For this review, use the dimensioned drawing (mm, ordinates from the lowest corner) and the shaded views. A direction names the side the tool comes from. Give positions to 0.01 mm unless a question says otherwise; leave off trailing zeros. Write each loop counter-clockwise with the first axis right and the second up, starting at its lowest first coordinate (ties: lowest second). Pieces come first, ordered by that corner, then holes. Notation, with made-up numbers: (-10, 62) -> (33, 62) arc R16 ccw to (33, 87) -> close; hole circle Ø4 at (61, 21). An arc over 180 degrees is marked (long way). Answer as CSV lines item,"result".
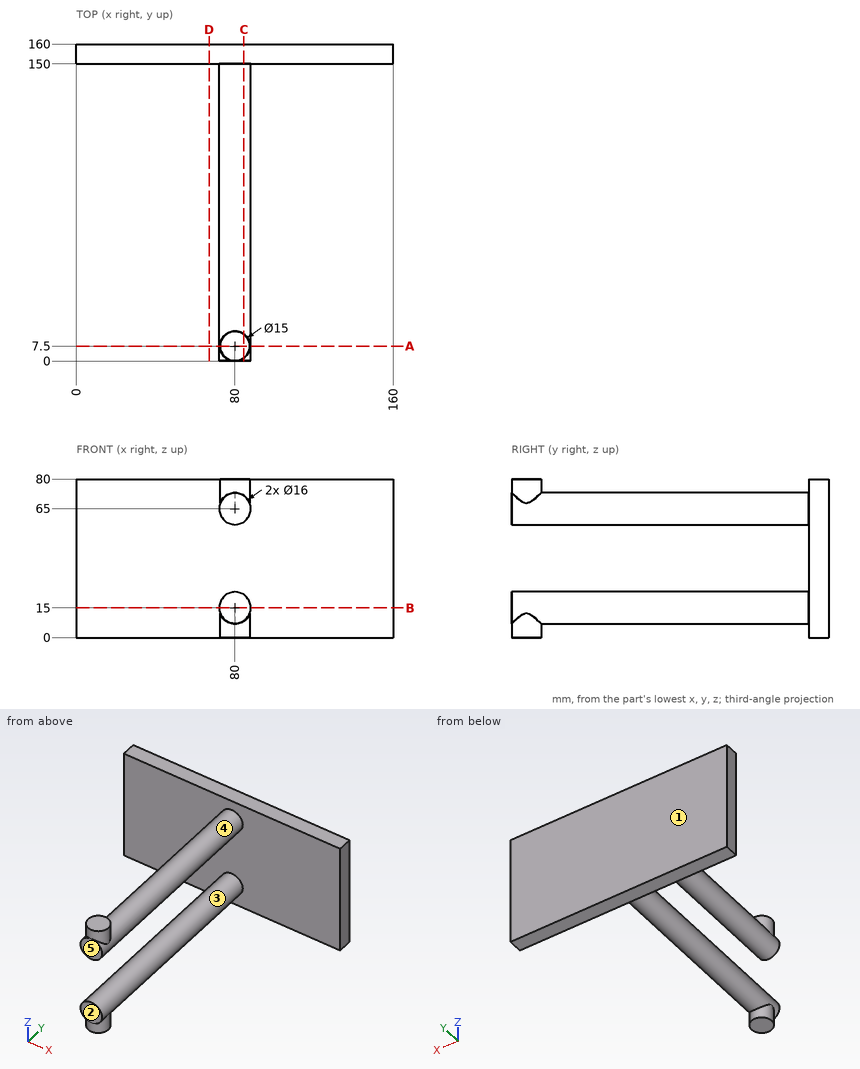
Q1. Clearance check with flat-ended pins moving along their axes: pin 1 (8 mm diameter, centred on x = 100, z = 47, fed in from -Y); pin 2 (1 mm diameter, centred on x = 85, y = 106, fed in from +Z); pin 3 (4 mm diameter, centred on y = 105.5, z = 58, fed in from -X) (3 decimals). State where each tip first meets the part, or that it passes through.
Answer block:
pin 1,"stops at y = 150"
pin 2,"stops at z = 71.61"
pin 3,"stops at x = 73.755"
Q2. Draft analysis for pull direction Y (two halves, no side actions). For the marked faces 1, 2 and 3, state which applies: released by +Y, released by -Y, zero draft, split by the parting line, or undercut.
Answer block:
face 1,"released by +Y"
face 2,"released by -Y"
face 3,"undercut"
Q3. Add section C-C (x = 84.5). Write out the cut boundary in (y, z).
Answer block:
outline,"(0, 8.39) -> (1.5, 8.39) -> (1.5, 0) -> (13.5, 0) -> (13.5, 8.39) -> (150, 8.39) -> (150, 0) -> (160, 0) -> (160, 80) -> (150, 80) -> (150, 71.61) -> (13.5, 71.61) -> (13.5, 80) -> (1.5, 80) -> (1.5, 71.61) -> (0, 71.61) -> (0, 58.39) -> (150, 58.39) -> (150, 21.61) -> (0, 21.61) -> close"
Q4. Add section D-D (x = 67). Write out the cut boundary in (y, z), plus the area to 3 significant figures.
Answer block:
outline,"(150, 0) -> (160, 0) -> (160, 80) -> (150, 80) -> close"
area,"800 mm2"
Q5. For the marked faces 4 and 5, list the 3-axis set-ups (+Z, -Z, +X, -X, +Y, -Y) from which the entire face can be reached by the end or side of a thin tool; tool diameter is ignored.
Answer block:
face 4,"none"
face 5,"+Z, -Z, +X, -X, -Y"
Q6. Add section B-B (z = 15). Write out the cut boundary in (x, y), plus the area to 3 significant figures.
Answer block:
outline,"(0, 150) -> (72, 150) -> (72, 0) -> (88, 0) -> (88, 150) -> (160, 150) -> (160, 160) -> (0, 160) -> close"
area,"4,000 mm2"
Q7. Add section A-A (y = 7.5). Write out the cut boundary in (x, z), plus the area to 3 significant figures.
Answer block:
outline,"(72.5, 0) -> (87.5, 0) -> (87.5, 12.22) arc R8 ccw (long way) to (72.5, 12.22) -> close; (72.5, 67.78) arc R8 ccw (long way) to (87.5, 67.78) -> (87.5, 80) -> (72.5, 80) -> close"
area,"655 mm2"
Q8. To check wall thickness, follow probe 1 along Y at (x, z) = (116, 26); probe 2 along X at (y, z) = (31.5, 67); probe 3 along X at (y, z) = (79, 66). State the ranges of each line that lie inside material, in increasing order. Write a range as [from, to].
Answer block:
probe 1,"y = [150, 160]"
probe 2,"x = [72.25, 87.75]"
probe 3,"x = [72.06, 87.94]"
